Geometry check sheet. Reference: the model listing, model coordinates, mm. Face numbers are marked on the shaded views. A direction names the side the tool comes from. Give positions to 0.01 mm unless a question says otherwise; leave off trailing zeros. Loops run counter-clockwise (first coordinate to the right, second up) from the corner with the lowest first, then second, coordinate; pieces in that order, holes last. Notation, with made-up numbers: (-29, 48) - (-18, 48) arc R9 cw to (-18, 64) - close; hole circle Ø9 at (25, -6.5). An arc over 180 degrees is marked (long way). One line per question, with ' | ' between items. Start each with the question number.
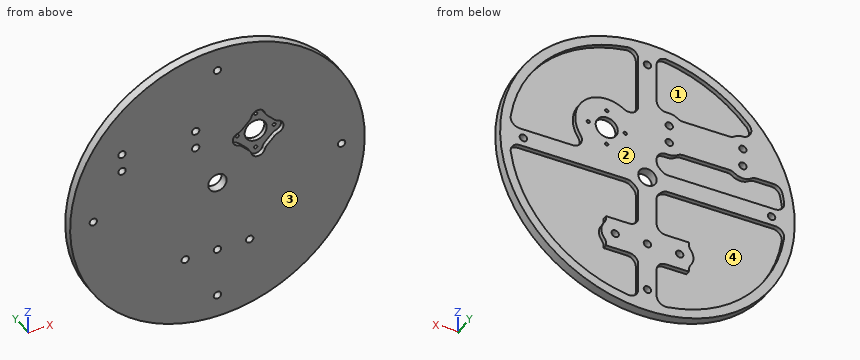
from build123d import *

# Parameters (mm, degrees)
SKETCH3_R                   = 101.6
BOSS_EXTRUDE1_DEPTH         = 6.35
SKETCH4_R                   = 7.620000000000008
CUT_EXTRUDE1_DEPTH          = 144.82434599190776
F_1_4_20_TAPPED_HOLE5_D     = 5.1054
F_1_4_20_TAPPED_HOLE5_DEPTH = 19.05
F_1_4_20_TAPPED_HOLE5_TIP   = 1.5338169021916532
CUT_EXTRUDE2_DEPTH          = 3.175
F_1_4_20_TAPPED_HOLE2_D     = 5.1054
F_1_4_20_TAPPED_HOLE2_DEPTH = 19.05
F_1_4_20_TAPPED_HOLE2_TIP   = 1.5338169021916532
F_1_4_20_TAPPED_HOLE4_D     = 5.1054
F_1_4_20_TAPPED_HOLE4_DEPTH = 19.05
F_1_4_20_TAPPED_HOLE4_TIP   = 1.5338169021916532
FILLET3_R                   = 6.35
F_4_40_TAPPED_HOLE1_D       = 2.2606
CUT_EXTRUDE3_DEPTH          = 3.175
FILLET4_R                   = 6.35


with BuildPart() as part:
    # Sketch3 → Boss-Extrude1 (new body)
    with BuildSketch(Plane(origin=(0, 0, 0), x_dir=(1, 0, 0), z_dir=(0, 1, 0))):
        with Locations(Location((0, 0, 0), (0, 0, 270))):
            Circle(SKETCH3_R)
    extrude(amount=BOSS_EXTRUDE1_DEPTH)

    # Sketch4 → Cut-Extrude1 (cut, through all)
    with BuildSketch(Plane(origin=(0, 6.35, 0), x_dir=(1, 0, 0), z_dir=(0, 1, 0))):
        with BuildLine():
            ThreePointArc((2.703e-14, -6.349999999999998), (4.490128060534583, -4.490128060534569), (6.349999999999998, -1.56e-15))
            Line((6.349999999999994, 0), (0, 0))
            Line((0, 0), (0, -6.349999999999994))
        make_face()
        with BuildLine():
            Line((0, 0), (6.349999999999994, 0))
            ThreePointArc((6.349999999999998, 0), (-4.490128060534585, 4.490128060534566), (2.703e-14, -6.349999999999998))
            Line((0, -6.349999999999994), (0, 0))
        make_face()
        with Locations(Location((28.06330037834144, -28.063300378340767, 0), (0, 0, 270))):
            Circle(SKETCH4_R)
    extrude(amount=-CUT_EXTRUDE1_DEPTH, mode=Mode.SUBTRACT)

    # 1/4-20 Tapped Hole5
    with Locations(Plane(origin=(0, 6.35, -85.599778), x_dir=(0, 0, 1), z_dir=(0, 1, 0))):
        with Locations((0, 0), (85.599778, -85.599778), (171.199556, 0), (85.599778, 85.599778)):
            Hole(F_1_4_20_TAPPED_HOLE5_D / 2, depth=F_1_4_20_TAPPED_HOLE5_DEPTH)
            with Locations((0, 0, -(F_1_4_20_TAPPED_HOLE5_DEPTH + F_1_4_20_TAPPED_HOLE5_TIP / 2))):  # 118° drill point
                Cone(0, F_1_4_20_TAPPED_HOLE5_D / 2, F_1_4_20_TAPPED_HOLE5_TIP, mode=Mode.SUBTRACT)

    # Sketch6 → Cut-Extrude2 (cut)
    with BuildSketch(Plane(origin=(0, 6.35, 0), x_dir=(1, 0, 0), z_dir=(0, 1, 0))):
        with BuildLine():
            Line((-28.575000000000006, 61.9125), (-6.349999999999998, 61.912500000000016))
            Line((-6.349999999999998, 61.912500000000016), (-6.350000000000037, 95.03809762405811))
            ThreePointArc((-6.350000000000033, 95.03809762405811), (-67.35192090801853, 67.35192090801877), (-95.03809762405808, 6.350000000000408))
            Line((-95.03809762405807, 6.350000000000351), (-10.998522628062574, 6.349999999999822))
            ThreePointArc((-10.998522628062497, 6.349999999999779), (-8.980256121069209, 8.980256121069099), (-6.349999999999914, 10.99852262806242))
            Line((-6.349999999999998, 10.99852262806245), (-6.349999999999998, 39.687499999999986))
            Line((-6.349999999999998, 39.687499999999986), (-28.575, 39.687499999999986))
            Line((-28.575, 39.687499999999986), (-28.575, 43.70048417143843))
            ThreePointArc((-28.575000000000216, 43.700484171438355), (-31.750000000000014, 50.80000000000001), (-28.57500000000022, 57.89951582856166))
            Line((-28.575000000000006, 57.89951582856159), (-28.575000000000006, 61.9125))
        make_face()
        with BuildLine():
            Line((6.350000000002216, 95.03809762405781), (6.349999999999998, 61.91250000000002))
            Line((6.349999999999998, 61.91250000000002), (28.575000000000028, 61.91250000000004))
            Line((28.575000000000028, 61.91250000000004), (28.575000000000028, 57.89951582856217))
            ThreePointArc((28.574999999999754, 57.89951582856208), (31.75000000000002, 50.80000000000001), (28.57499999999976, 43.700484171437935))
            Line((28.575000000000035, 43.70048417143784), (28.575000000000035, 39.687499999999986))
            Line((28.575000000000035, 39.687499999999986), (6.349999999999998, 39.687499999999986))
            Line((6.349999999999998, 39.687499999999986), (6.349999999999998, 10.998522628062325))
            ThreePointArc((6.350000000000048, 10.998522628062343), (8.980256121069322, 8.980256121068983), (10.998522628062583, 6.349999999999632))
            Line((10.998522628062709, 6.349999999999706), (95.03809762405771, 6.350000000002941))
            ThreePointArc((95.03809762405791, 6.3500000000029555), (67.35192090801839, 67.35192090801893), (6.350000000002218, 95.03809762405797))
        make_face()
        with BuildLine():
            ThreePointArc((-6.349999999999907, -10.998522628062423), (-8.980256121069205, -8.9802561210691), (-10.9985226280625, -6.349999999999777))
            Line((-10.998522628062572, -6.349999999999824), (-95.03809762405797, -6.350000000001099))
            ThreePointArc((-95.03809762405804, -6.350000000001103), (-93.90381775371628, -15.957302756946103), (-91.8008850719861, -25.399999999999988))
            Line((-91.8008850719861, -25.400000000000006), (-72.9109158285621, -25.400000000000006))
            ThreePointArc((-72.91091582856204, -25.400000000000183), (-65.81140000000006, -22.22499999999998), (-58.71188417143806, -25.400000000000126))
            Line((-58.71188417143801, -25.400000000000084), (-22.110915828561872, -25.400000000000006))
            ThreePointArc((-22.110915828561865, -25.400000000000006), (-18.899964966668318, -23.054904399605476), (-15.011400000000005, -22.22499999999998))
            Line((-15.011400000000005, -22.22499999999998), (-6.349999999999998, -22.22499999999998))
            Line((-6.349999999999998, -22.22499999999998), (-6.349999999999998, -10.998522628062457))
        make_face()
        with BuildLine():
            Line((95.03809762405827, -6.349999999998817), (28.063300378341538, -6.350000000000001))
            ThreePointArc((28.063300378341545, -6.350000000000005), (43.41692231780658, -43.416922317805984), (6.35000000000068, -28.063300378340763))
            Line((6.350000000000339, -28.063300378340763), (6.3500000000001044, -95.03809762405808))
            ThreePointArc((6.350000000000042, -95.03809762405811), (67.35192090801905, -67.35192090801824), (95.0380976240582, -6.349999999998817))
        make_face()
        with BuildLine():
            Line((-65.81140000000002, -53.97499999999998), (-78.48096504885757, -53.97499999999998))
            ThreePointArc((-78.48096504885758, -53.97499999999996), (-47.123429994015716, -82.77647519433948), (-6.350000000001006, -95.03809762405804))
            Line((-6.350000000000966, -95.03809762405798), (-6.349999999999998, -53.97499999999998))
            Line((-6.349999999999998, -53.97499999999998), (-15.011400000000005, -53.97499999999998))
            ThreePointArc((-15.011400000000007, -53.97499999999998), (-18.8999649666683, -53.14509560039449), (-22.11091582856184, -50.79999999999998))
            Line((-22.110915828561843, -50.79999999999998), (-58.71188417143799, -50.799999999999876))
            ThreePointArc((-58.71188417143805, -50.79999999999983), (-61.92283503333163, -53.14509560039445), (-65.81140000000002, -53.97499999999998))
        make_face()
    extrude(amount=-CUT_EXTRUDE2_DEPTH, mode=Mode.SUBTRACT)

    # 1/4-20 Tapped Hole2
    with Locations(Plane(origin=(-22.225, 6.35, -50.8), x_dir=(0, 0, 1), z_dir=(0, 1, 0))):
        with Locations((0, 0), (0, 44.45), (0, 22.225)):
            Hole(F_1_4_20_TAPPED_HOLE2_D / 2, depth=F_1_4_20_TAPPED_HOLE2_DEPTH)
            with Locations((0, 0, -(F_1_4_20_TAPPED_HOLE2_DEPTH + F_1_4_20_TAPPED_HOLE2_TIP / 2))):  # 118° drill point
                Cone(0, F_1_4_20_TAPPED_HOLE2_D / 2, F_1_4_20_TAPPED_HOLE2_TIP, mode=Mode.SUBTRACT)

    # 1/4-20 Tapped Hole4
    with Locations(Plane(origin=(-65.8114, 6.35, 31.75), x_dir=(0, 0, 1), z_dir=(0, 1, 0))):
        with Locations((0, 0), (12.7, 0), (12.7, 50.8), (0, 50.8)):
            Hole(F_1_4_20_TAPPED_HOLE4_D / 2, depth=F_1_4_20_TAPPED_HOLE4_DEPTH)
            with Locations((0, 0, -(F_1_4_20_TAPPED_HOLE4_DEPTH + F_1_4_20_TAPPED_HOLE4_TIP / 2))):  # 118° drill point
                Cone(0, F_1_4_20_TAPPED_HOLE4_D / 2, F_1_4_20_TAPPED_HOLE4_TIP, mode=Mode.SUBTRACT)

    # Fillet3
    fillet3_edges = [part.edges().sort_by_distance(p)[0] for p in [
        (-10.998522628062535, 4.762499999999999, 6.349999999999799),
        (-6.349999999999952, 4.762499999999999, 10.998522628062439),
        (-6.3500000000009855, 4.762499999999999, 95.038097624058),
        (-95.03809762405801, 4.762499999999999, 6.350000000001101),
        (95.03809762405824, 4.762499999999999, 6.349999999998815),
        (6.350000000000073, 4.762499999999999, 95.0380976240581),
        (95.03809762405783, 4.762499999999999, -6.350000000002949),
        (10.998522628062645, 4.762499999999999, -6.349999999999669),
        (6.350000000000022, 4.762499999999999, -10.998522628062334),
        (6.349999999999998, 4.762499999999999, -39.687499999999986),
        (6.349999999999998, 4.762499999999999, -61.91250000000002),
        (6.35000000000222, 4.762499999999999, -95.0380976240579),
        (-6.350000000000035, 4.762499999999999, -95.03809762405811),
        (-95.03809762405808, 4.762499999999999, -6.350000000000376),
        (-10.998522628062535, 4.762499999999999, -6.349999999999801),
        (-6.349999999999955, 4.762499999999999, -10.998522628062435),
        (-6.349999999999998, 4.762499999999999, -39.687499999999986),
        (28.06330037834154, 4.762499999999999, 6.350000000000007),
        (6.350000000000506, 4.762499999999999, 28.06330037834077),
        (-6.349999999999998, 4.762499999999999, -61.912500000000016),
        (-72.91091582856207, 4.762499999999999, 25.400000000000095),
        (-58.71188417143803, 4.762499999999999, 25.400000000000105),
        (-22.110915828561843, 4.762499999999999, 50.79999999999998),
        (-22.11091582856187, 4.762499999999999, 25.400000000000006),
        (-28.575000000000117, 4.762499999999999, -57.899515828561626),
        (-28.57500000000011, 4.762499999999999, -43.70048417143839),
        (28.574999999999896, 4.762499999999999, -43.70048417143789),
        (28.57499999999989, 4.762499999999999, -57.89951582856213),
        (-91.80088507198612, 4.762499999999999, 25.399999999999995),
        (-58.711884171438015, 4.762499999999999, 50.799999999999855),
        (-78.48096504885758, 4.762499999999999, 53.97499999999998),
        (-6.349999999999998, 4.762499999999999, 22.22499999999998),
        (-6.349999999999998, 4.762499999999999, 53.97499999999998),
    ]]
    fillet(fillet3_edges, radius=FILLET3_R)

    # #4-40 Tapped Hole1 (through all)
    with Locations(Plane(origin=(28.063300378, 6.35, 15.335360378), x_dir=(0, 0, 1), z_dir=(0, 1, 0))):
        with Locations((0, 0), (12.72794, -12.72794), (25.45588, 0), (12.72794, 12.72794)):
            Hole(F_4_40_TAPPED_HOLE1_D / 2)

    # Sketch15 → Cut-Extrude3 (cut)
    with BuildSketch(Plane.XZ):
        with BuildLine():
            Line((40.79124037834144, 23.300800378340764), (32.82580037834144, 15.335360378340768))
            ThreePointArc((32.82580037834144, 15.335360378340768), (28.06330037834144, 10.572860378340765), (23.30080037834144, 15.335360378340768))
            Line((23.30080037834144, 15.335360378340768), (15.335360378341441, 23.300800378340767))
            ThreePointArc((15.335360378341441, 23.300800378340767), (10.572860378341442, 28.063300378340767), (15.335360378341441, 32.825800378340766))
            Line((15.335360378341441, 32.825800378340766), (23.30080037834144, 40.79124037834077))
            ThreePointArc((23.30080037834144, 40.79124037834077), (28.06330037834144, 45.55374037834076), (32.82580037834144, 40.79124037834077))
            Line((32.82580037834144, 40.79124037834077), (40.79124037834144, 32.82580037834077))
            ThreePointArc((40.79124037834144, 32.82580037834077), (45.553740378341445, 28.063300378340767), (40.79124037834144, 23.300800378340764))
        make_face()
    extrude(amount=-CUT_EXTRUDE3_DEPTH, mode=Mode.SUBTRACT)

    # Fillet4
    fillet4_edges = [part.edges().sort_by_distance(p)[0] for p in [
        (23.30080037834144, 1.5875, 40.79124037834077),
        (15.335360378341441, 1.5875, 32.825800378340766),
        (15.335360378341441, 1.5875, 23.300800378340767),
        (23.300800378341435, 1.5875, 15.335360378340768),
        (32.82580037834144, 1.5875, 15.335360378340768),
        (40.79124037834144, 1.5875, 23.300800378340767),
        (40.79124037834144, 1.5875, 32.82580037834077),
        (32.82580037834144, 1.5875, 40.79124037834077),
    ]]
    fillet(fillet4_edges, radius=FILLET4_R)


solid = part.part
(1) Section check C-C, the plane y = 2. Count the separate pieces of the cut face and the enclosed holes in it, and give its area (3 significant figures).
(2) Section check D-D, the plane z = -75.5. Record the boundary of the cut face in (x, y) (3 decimals).
(3) Mould release check, pull along X, two halves, no side actions. Record for the marked faces 3 and 4: pulls with the +X half, pulls with the -X half, needs draft (parallel to the pull), parting line crosses it, or undercut.
(4) Tool access check on the marked faces 1 and 2. Record the directions out of +Z, -Z, +X, -X, +Y, -Y that give a thin tool (end or side, any length) a straight path to the whole face; none if there is none.
(5) Depth check by flat-ended pin: pin 1 Ø3 at (x, z) = (-49.5, 27.5) entering from -Y; pin 2 Ø2 at (y, z) = (3.5, -17) entering from +X; pin 3 Ø0.8 at (y, z) = (4.5, -61) entering from +X; pin 4 Ø1.6 at (y, z) = (5.5, 78.5) entering from +X. Enter the tip coordinate at first touch or a pass-through.
(6) Section check A-A, the plane x = 0. Record the boundary of the cut face in (y, z), and give its area (3 significant figures).
(7) Material ranges on line 1 (X direction, y = 5.25, z = -26.5); line 2 (Z direction, x = 37.5, y = 3.5); line 3 (X direction, y = 3.75, z = -7), recorded low to high.
(8) Section check B-B, the plane z = 0. Record the boundary of the cut face in (x, y).
Numbers:
1) separate pieces: 1 | enclosed holes: 13 | area: 31,400 mm^2
2) outline: (-67.988, 0) - (67.988, 0) - (67.988, 6.35) - (58.072, 6.35) - (58.072, 3.175) - (6.35, 3.175) - (6.35, 6.35) - (-6.35, 6.35) - (-6.35, 3.175) - (-58.072, 3.175) - (-58.072, 6.35) - (-67.988, 6.35) - close
3) face 3: needs draft | face 4: undercut
4) face 1: +Y | face 2: +Z, -Z, +X, -X, +Y
5) pin 1: y = 0 | pin 2: x = 100.33 | pin 3: x = 81.55 | pin 4: x = 65.46
6) outline: (0, -101.6) - (6.35, -101.6) - (6.35, -88.15) - (0, -88.15) - close; (0, -83.05) - (6.35, -83.05) - (6.35, -53.35) - (0, -53.35) - close; (0, -48.25) - (6.35, -48.25) - (6.35, -6.35) - (0, -6.35) - close; (0, 6.35) - (6.35, 6.35) - (6.35, 83.05) - (0, 83.05) - close; (0, 88.15) - (6.35, 88.15) - (6.35, 101.6) - (0, 101.6) - close | area: 1,110 mm^2
7) line 1: -98.08 to -91.49, -6.35 to 6.35, 91.49 to 98.08 | line 2: -94.43 to -87.56, -6.35 to 47.62, 87.56 to 94.43 | line 3: -101.36 to -90.79, -11.4 to 11.4, 90.79 to 101.36
8) outline: (-101.6, 0) - (-88.15, 0) - (-88.15, 6.35) - (-101.6, 6.35) - close; (-83.05, 0) - (-6.35, 0) - (-6.35, 6.35) - (-83.05, 6.35) - close; (6.35, 0) - (83.05, 0) - (83.05, 6.35) - (6.35, 6.35) - close; (88.15, 0) - (101.6, 0) - (101.6, 6.35) - (88.15, 6.35) - close
